Autodesk Inventor part; units mm, degrees
ref_plane "YZ Plane" through (0, 0, 0) normal (1, 0, 0) x (0, 1, 0)
ref_plane "XZ Plane" through (0, 0, 0) normal (0, 1, 0) x (-1, 0, 0)
ref_plane "XY Plane" through (0, 0, 0) normal (0, 0, 1) x (1, 0, 0)
sketch "Эскиз1" plane through (0, 0, 0) normal (0, 0, 1) x (1, 0, 0)
  line L0 (15, -22.25) -> (15, 22.25)
  line L1 (15, 22.25) -> (-20, 22.25)
  line L2 (-20, 22.25) -> (-20, -22.25)
  line L3 (-20, -22.25) -> (15, -22.25)
  circle A0 centre (8.763, 2.3275) radius 1.5
  circle A1 centre (8.763, 7.3275) radius 1.5
  circle A2 centre (-11.237, -7.6725) radius 1.5
  circle A3 centre (-11.237, -2.6725) radius 1.5
  circle A4 centre (8.763, -2.6725) radius 1.5
  circle A5 centre (8.763, -7.6725) radius 1.5
  circle A6 centre (-11.237, 2.3275) radius 1.5
  circle A7 centre (-11.237, 7.3275) radius 1.5
  line L4 (-25, 92.25) -> (-62.0049, 92.25)
  line L5 (-103.637, 92.25) -> (-67.893, 92.25)
  circle A8 centre (-49, 104.25) radius 1.5
  circle A9 centre (-42, 104.25) radius 1.5
  circle A10 centre (-35, 104.25) radius 1.5
  circle A11 centre (-35, 111.25) radius 1.5
  circle A12 centre (-42, 118.25) radius 1.5
  circle A13 centre (-49, 118.25) radius 1.5
  circle A14 centre (-49, 111.25) radius 1.5
  circle A15 centre (-35, 118.25) radius 1.5
  circle A16 centre (-42, 111.25) radius 1.5
  circle A17 centre (-42, 97.25) radius 1.5
  circle A18 centre (-35, 97.25) radius 1.5
  circle A19 centre (-49, 97.25) radius 1.5
  line L6 (-25, 92.25) -> (-62.0049, 92.25)
  line L7 (-25, 95.25) -> (-25, 92.25)
  line L8 (-20, 95.25) -> (-25, 95.25)
  line L9 (-20, 95.25) -> (-20, 123.25)
  line L10 (-28, 123.25) -> (-20, 123.25)
  line L11 (-28, 129.25) -> (-28, 123.25)
  line L12 (-28, 129.25) -> (-62.0049, 129.25)
  line L13 (-62.0049, 92.25) -> (-62.0049, 129.25)
  line L14 (-5.1452, 11.625) -> (-40, 100) construction
  arc A20 (-32.5697, 102.9649) -> (-47.4303, 97.0351) centre (-40, 100) ccw
  line L15 (-5.1452, 11.625) -> (-22.5726, 55.8125) construction
  arc A21 (-13.8135, 8.0713) -> (-4.3725, 15.1785) centre (-0.8009, 0.6099) ccw
  line L16 (12.7625, 7.0157) -> (-32.7662, 103.4164)
  line L17 (-47.6184, 97.5588) -> (-15.0854, -3.9674)
  point P0 (0, 0)
  point P1 (-13.8589, 33.7187)
  point P2 (-33.6095, 104.8127)
  point P3 (-34.2206, 105.5316)
  point P4 (-47.7749, 98.1155)
  point P5 (-47.5011, 97.1926)
  dimension "d0" = 8
  dimension "d1" = 95
  dimension "d2" = 100
  dimension "d3" = 40
  dimension "d4" = 15
extrude "Выдавливание1" add sketch "Эскиз1" along normal blind 3 contours L16 A21 L17 L2 L1 | L1 L2 L17 L4 L16 | L4 L17 A19 A20 A10 L16 | A20 A10 | A10 A20 | A1 | A2 | A3 | A4 | A5 | A7 | A9
sketch "Эскиз2" plane through (0, 0, 3) normal (0, 0, 1) x (1, 0, 0)
  circle A0 centre (-38.5661, 86.5462) radius 1.5
  line L0 (-47.5011, 97.1926) -> (-15.0854, -3.9674)
  circle A1 centre (-35.5146, 77.0232) radius 1.5
  circle A2 centre (-32.463, 67.5001) radius 1.5
  circle A3 centre (-29.4114, 57.9771) radius 1.5
  circle A4 centre (-26.3599, 48.4541) radius 1.5
  circle A5 centre (-23.3083, 38.9311) radius 1.5
  circle A6 centre (-20.2568, 29.408) radius 1.5
  circle A7 centre (-17.2052, 19.885) radius 1.5
  circle A8 centre (-42, 97.25) radius 1.5
  circle A9 centre (-11.237, 2.3275) radius 1.5
  point P0 (0, 0)
  dimension "d7" = 3
  dimension "d10" = 10
  dimension "d17" = 5.2562
  dimension "d18" = 5.26
extrude "Выдавливание2" cut sketch "Эскиз2" against normal blind 3 contours A0 | A1 | A2 | A3 | A4 | A5 | A6 | A7
sketch "Эскиз3" plane through (0, 0, 3) normal (0, 0, 1) x (1, 0, 0)
  circle A0 centre (-35, 97.25) radius 1.5
  line L0 (12.7625, 7.0157) -> (-32.7662, 103.4164)
  circle A1 centre (-30.5318, 87.7899) radius 1.5
  circle A2 centre (-26.2613, 78.7476) radius 1.5
  circle A3 centre (-21.9908, 69.7054) radius 1.5
  circle A4 centre (-17.7202, 60.6631) radius 1.5
  circle A5 centre (-13.4497, 51.6208) radius 1.5
  circle A6 centre (-9.1792, 42.5786) radius 1.5
  circle A7 centre (-4.9086, 33.5363) radius 1.5
  circle A8 centre (-0.6381, 24.494) radius 1.5
  point P0 (0, 0)
  dimension "d19" = 3
  dimension "d20" = 4.6533
  dimension "d21" = 4.653
  dimension "d24" = 10
extrude "Выдавливание3" cut sketch "Эскиз3" against normal blind 3 contours A1 | A2 | A3 | A4 | A5 | A6 | A7 | A8
properties part number "ЛЦМК000002.00.00.00.00.19 мост"
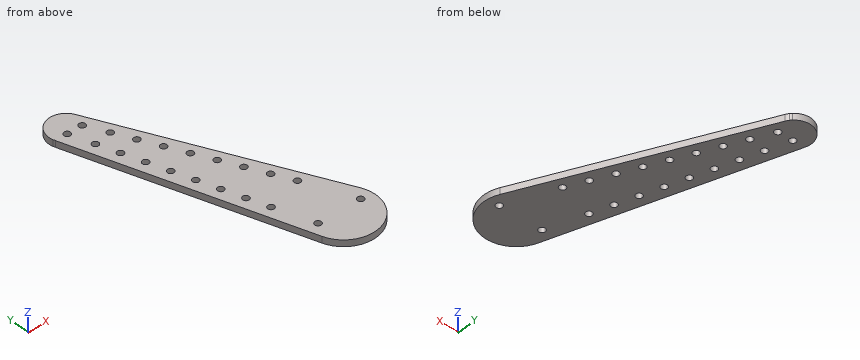
The model under review builds one solid part; all positions refer to its coordinate system, in mm. Round coordinates to 2 decimals unless told otherwise and drop trailing zeros. Order: outer loops, then holes, each group sorted by start corner. A loop starts at its lowest first (then second) coordinate and runs counter-clockwise, first axis right, second up.
(1) Take a section at A-A, the plane x = -26. State the section outline as (y, z) points, plus the area to 3 significant figures.
Working result:
outline: (30.09, 0) - (47, 0) - (47, 3) - (30.09, 3) - close; (49.91, 0) - (77.27, 0) - (77.27, 3) - (49.91, 3) - close; (80.22, 0) - (89.09, 0) - (89.09, 3) - (80.22, 3) - close
area: 159 mm2
(2) For P1, Ø1.5, axis at x = -2, z = 1, coming from the +Y side, flat-tipped, find the tip position at first contact; note if it passes through.
Working result:
P1: stops at y = 39.86
(3) Take a section at D-D, the plane y = 83.5. State the section outline as (x, z) points, plus the area to 3 significant figures.
Working result:
outline: (-43.11, 0) - (-23.36, 0) - (-23.36, 3) - (-43.11, 3) - close
area: 59.3 mm2
(4) Take a section at B-B, the plane z = 2.4. Count the separate pieces of the cut face and the enclosed holes in it, plus the area to 3 significant figures.
Working result:
separate pieces: 1
enclosed holes: 20
area: 2,780 mm2
(5) Take a section at C-C, the plane x = -42. State the section outline as (y, z) points, plus the area to 3 significant figures.
Working result:
outline: (80.03, 0) - (95.75, 0) - (95.75, 3) - (80.03, 3) - close; (98.75, 0) - (107.75, 0) - (107.75, 3) - (98.75, 3) - close
area: 74.2 mm2
(6) Wall thickness on L1, parallel to X at y = 3.5, z = 2.6; L2, parallel to X at y = 47.5, z = 0.7; L3, parallel to Y at x = -12.5, z = 1.55: over which ranges is each line inside the solid? List them lowest first.
Working result:
L1: x = -17.48 to -12.17, -10.3 to 7.83, 9.7 to 13.92
L2: x = -31.58 to -27.52, -25.2 to -6.36
L3: y = -8.78 to 1.52, 3.14 to 50.46, 52.78 to 60.51
